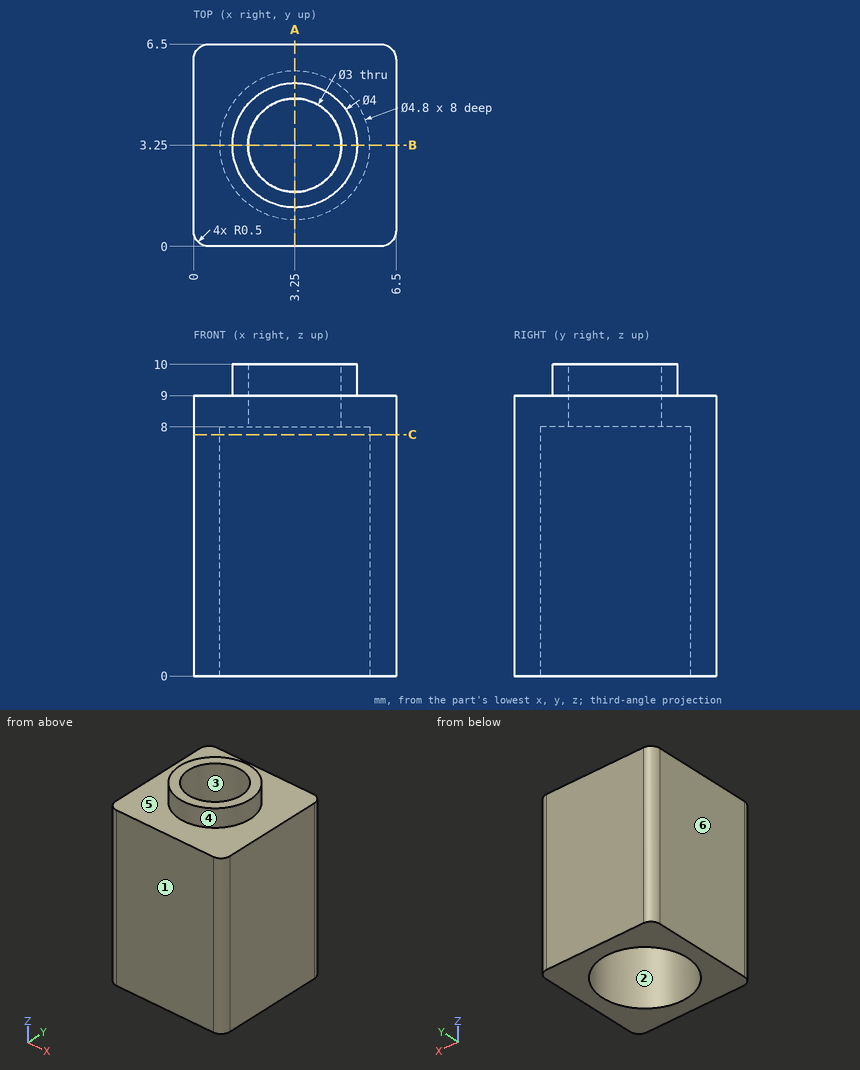
Could you check a few things on this drawing? It's one solid part, dimensions in mm from its lowest x, y, z. A direction names the side the tool comes from. Coordinates: 2 decimals unless noted, no trailing zeros. Write each loop counter-clockwise with the first axis right and the second up, starting at its lowest first coordinate (ties: lowest second). Pieces come first, ordered by that corner, then holes.
Q1. Which directions (+Z, -Z, +X, -X, +Y, -Y) give clear straight access to the entire face, cutting with the end or side of a thin tool? Please do the marked faces 5 and 6.
Results found:
face 5: +Z
face 6: +Z, -Z, -X, +Y, -Y
Q2. Imagine slicing it at A-A, the plane x = 3.25. List the corners of the cut face in (y, z) for me, plus the area to 3 significant figures.
Results found:
outline: (0, 0) - (0.85, 0) - (0.85, 8) - (1.75, 8) - (1.75, 10) - (1.25, 10) - (1.25, 9) - (0, 9) - close; (4.75, 8) - (5.65, 8) - (5.65, 0) - (6.5, 0) - (6.5, 9) - (5.25, 9) - (5.25, 10) - (4.75, 10) - close
area: 18.1 mm2
Q3. Please list where these lines run through material, in increasing order: L1, parallel to X at y = 3.25, z = 8.6; L2, parallel to Y at x = 3.25, z = 9.3; L3, parallel to Y at x = 3.25, z = 1.75.
Results found:
L1: x = 0 to 1.75, 4.75 to 6.5
L2: y = 1.25 to 1.75, 4.75 to 5.25
L3: y = 0 to 0.85, 5.65 to 6.5
Q4. Imagine slicing it at C-C, the plane z = 7.75. List the corners of the cut face in (x, y) for me, plus the area to 3 significant figures.
Results found:
outline: (0, 0.5) arc R0.5 ccw to (0.5, 0) - (6, 0) arc R0.5 ccw to (6.5, 0.5) - (6.5, 6) arc R0.5 ccw to (6, 6.5) - (0.5, 6.5) arc R0.5 ccw to (0, 6) - close; hole circle Ø4.8 at (3.25, 3.25)
area: 23.9 mm2
Q5. If we mould it in two halves opening along X, with no side actions, what happens to the marked faces 1, 2, 3 and 4? For each: +X half, -X half, draft (parallel to the pull), parting line (faces both ways), or undercut.
Results found:
face 1: draft
face 2: undercut
face 3: undercut
face 4: parting line
